Could you check a few things on this drawing? It's one solid part, dimensions in mm from its lowest x, y, z. Round coordinates to 2 decimals unless told otherwise and drop trailing zeros. Write each loop counter-clockwise with the first axis right and the second up, starting at its lowest first coordinate (ties: lowest second). Pieces come first, ordered by that corner, then holes. Notation, with made-up numbers: (79, 62.5) - (87, 62.5) arc R20 cw to (87, 92.5) - close; hole circle Ø10 at (-33, 83.25). An arc over 180 degrees is marked (long way). One line per question, with ' | ' between items. Start each with the question number.
(1) Imagine slicing it at D-D (y = 3.5). Write out the boundary of the cut face in (x, z).
(2) Imagine slicing it at B-B (y = 43). Write out the boundary of the cut face in (x, z).
(3) Will these pins go through, and if not, where does the flat tip stop? pin 1 (4 mm diameter, centred on y = 25.5, z = 6.5, fed in from +X); pin 2 (6 mm diameter, centred on y = 11.5, z = 8.5, fed in from -X); pin 3 (1.5 mm diameter, centred on x = 50, z = 7.5, fed in from -Y); pin 4 (4 mm diameter, centred on x = 63.5, z = 7.5, fed in from +Y).
(4) Imagine slicing it at C-C (z = 8). Write out the boundary of the cut face in (x, y), plus the area to 3 significant figures.
(5) If I drill on L1, parallel to Y at x = 94, z = 7.75; L2, parallel to Z at x = 87.5, y = 47.5; L3, parallel to X at y = 25, z = 9.5, over which ranges is the centre line in solid material (lowest first)?
(6) Imagine slicing it at A-A (x = 7.5). Write out the boundary of the cut face in (y, z), plus the area to 3 significant figures.
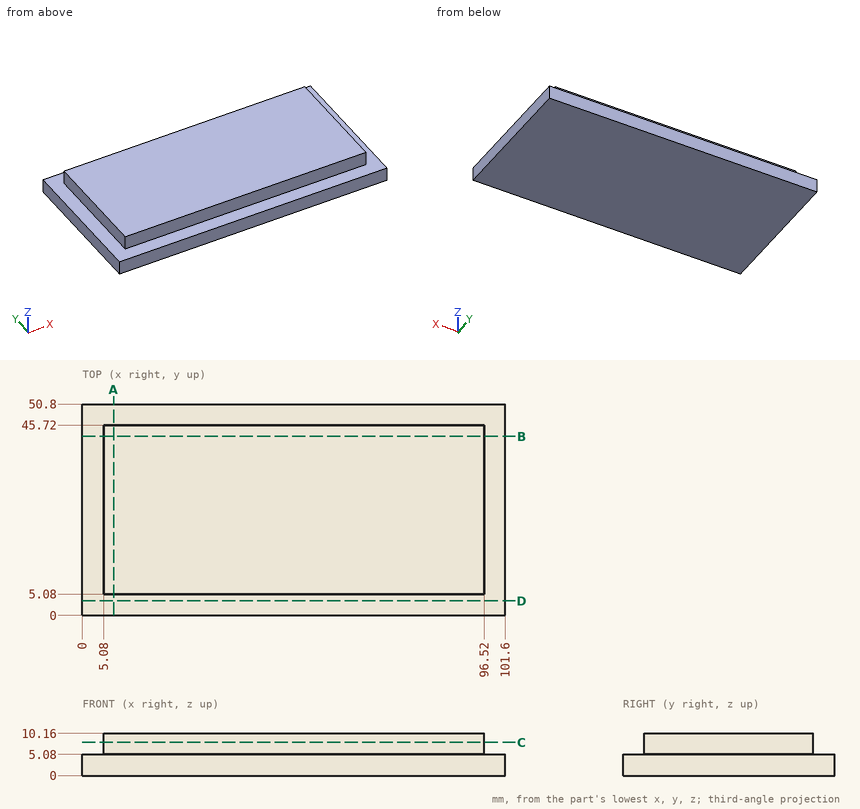
Check sheet entries:
1) outline: (0, 0) - (101.6, 0) - (101.6, 5.08) - (0, 5.08) - close
2) outline: (0, 0) - (101.6, 0) - (101.6, 5.08) - (96.52, 5.08) - (96.52, 10.16) - (5.08, 10.16) - (5.08, 5.08) - (0, 5.08) - close
3) pin 1: x = 101.6 | pin 2: x = 5.08 | pin 3: y = 5.08 | pin 4: y = 45.72
4) outline: (5.08, 5.08) - (96.52, 5.08) - (96.52, 45.72) - (5.08, 45.72) - close | area: 3,720 mm^2
5) L1: 5.08 to 45.72 | L2: 0 to 5.08 | L3: 5.08 to 96.52
6) outline: (0, 0) - (50.8, 0) - (50.8, 5.08) - (45.72, 5.08) - (45.72, 10.16) - (5.08, 10.16) - (5.08, 5.08) - (0, 5.08) - close | area: 465 mm^2
